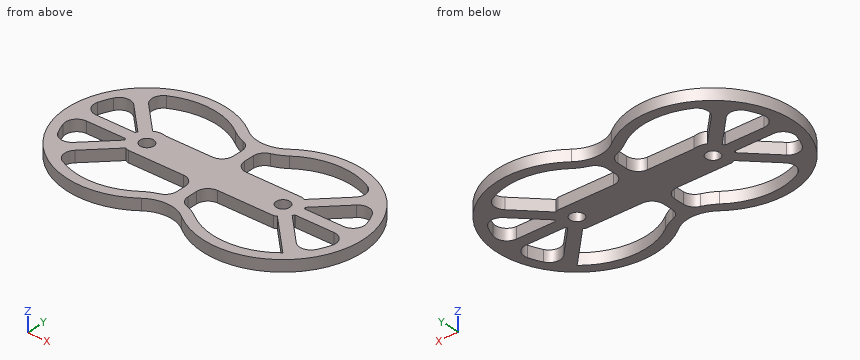
from build123d import *

# Parameters (mm, degrees)
SKETCH1_R           = 6
BOSS_EXTRUDE2_DEPTH = 10
FILLET2_R           = 10


with BuildPart() as part:
    # Sketch1 → Boss-Extrude2 (new body)
    with BuildSketch(Plane.XY):
        with BuildLine():
            ThreePointArc((-18.165151778, 55.726150839), (-130.527825355, 0), (-18.165151778, -55.726150839))
            ThreePointArc((-18.165151778, -55.726150839), (-0.527825355, -49.783359328), (17.109501067, -55.726150839))
            ThreePointArc((17.109501067, -55.726150839), (129.472174645, 0), (17.109501067, 55.726150839))
            ThreePointArc((17.109501067, 55.726150839), (-0.527825355, 49.783359328), (-18.165151778, 55.726150839))
        make_face()
        with Locations((-60.527825355, 0)):
            Circle(SKETCH1_R, mode=Mode.SUBTRACT)
        with Locations((59.472174645, 0)):
            Circle(SKETCH1_R, mode=Mode.SUBTRACT)
        with BuildLine():
            Line((-56.235975609, 14.912672635), (-5.527825355, 14.965504266))
            Line((-5.527825355, 14.965504266), (-5.527825355, 41.980686961))
            ThreePointArc((-5.527825355, 41.980686961), (-15.345309937, 44.512654742), (-24.210827936, 49.431643964))
            ThreePointArc((-24.210827936, 49.431643964), (-62.58583764, 61.303966527), (-100.078223296, 46.884728315))
            Line((-100.078223296, 46.884728315), (-67.337537784, 13.944016494))
            ThreePointArc((-67.337537784, 13.944016494), (-61.876707041, 15.459246345), (-56.235975609, 14.912672635))
        make_face(mode=Mode.SUBTRACT)
        with BuildLine():
            Line((-64.123905218, -15.095561897), (-5.527825355, -15.034512017))
            Line((-5.527825355, -15.034512017), (-5.527825355, -41.980686961))
            ThreePointArc((-5.527825355, -41.980686961), (-15.345309937, -44.512654742), (-24.210827936, -49.431643964))
            ThreePointArc((-24.210827936, -49.431643964), (-62.602390706, -61.303408593), (-100.103536918, -46.863362884))
            Line((-100.103536918, -46.863362884), (-67.345067046, -13.940336979))
            ThreePointArc((-67.345067046, -13.940336979), (-65.766427516, -14.607012931), (-64.123905218, -15.095561897))
        make_face(mode=Mode.SUBTRACT)
        with BuildLine():
            Line((-107.170792468, 39.835227443), (-74.430106955, 6.894515622))
            ThreePointArc((-74.430106955, 6.894515622), (-74.855512615, 5.960298411), (-75.218222877, 5))
            Line((-75.218222877, 5), (-121.6621997, 5))
            ThreePointArc((-121.6621997, 5), (-117.161402857, 23.559491206), (-107.170792468, 39.835227443))
        make_face(mode=Mode.SUBTRACT)
        with BuildLine():
            Line((-121.6621997, -5), (-75.218222877, -5))
            ThreePointArc((-75.218222877, -5), (-74.857121477, -5.956429468), (-74.433828207, -6.887006899))
            Line((-74.433828207, -6.887006899), (-107.192298079, -39.810032805))
            ThreePointArc((-107.192298079, -39.810032805), (-117.167762266, -23.544198292), (-121.6621997, -5))
        make_face(mode=Mode.SUBTRACT)
        with BuildLine():
            Line((4.472174645, 41.980686961), (4.472174645, 14.975923031))
            Line((4.472174645, 14.975923031), (63.304903434, 15.03721947))
            ThreePointArc((63.304903434, 15.03721947), (64.821395332, 14.56686711), (66.281887074, 13.944016494))
            Line((66.281887074, 13.944016494), (99.022572586, 46.884728315))
            ThreePointArc((99.022572586, 46.884728315), (61.530186929, 61.303966527), (23.155177226, 49.431643964))
            ThreePointArc((23.155177226, 49.431643964), (14.289659226, 44.512654742), (4.472174645, 41.980686961))
        make_face(mode=Mode.SUBTRACT)
        with BuildLine():
            Line((99.047886208, -46.863362884), (66.289416336, -13.940336979))
            ThreePointArc((66.289416336, -13.940336979), (64.962019266, -14.514454361), (63.586938832, -14.962502967))
            Line((63.586938832, -14.962502967), (4.472174645, -15.024093252))
            Line((4.472174645, -15.024093252), (4.472174645, -41.980686961))
            ThreePointArc((4.472174645, -41.980686961), (14.289659226, -44.512654742), (23.155177226, -49.431643964))
            ThreePointArc((23.155177226, -49.431643964), (61.546739995, -61.303408593), (99.047886208, -46.863362884))
        make_face(mode=Mode.SUBTRACT)
        with BuildLine():
            Line((106.136647368, -39.810032805), (73.378177497, -6.887006899))
            ThreePointArc((73.378177497, -6.887006899), (73.801470767, -5.956429468), (74.162572167, -5))
            Line((74.162572167, -5), (120.606548989, -5))
            ThreePointArc((120.606548989, -5), (116.112111556, -23.544198292), (106.136647368, -39.810032805))
        make_face(mode=Mode.SUBTRACT)
        with BuildLine():
            Line((120.606548989, 5), (74.162572167, 5))
            ThreePointArc((74.162572167, 5), (73.799861904, 5.960298411), (73.374456245, 6.894515622))
            Line((73.374456245, 6.894515622), (106.115141757, 39.835227443))
            ThreePointArc((106.115141757, 39.835227443), (116.105752147, 23.559491206), (120.606548989, 5))
        make_face(mode=Mode.SUBTRACT)
    extrude(amount=BOSS_EXTRUDE2_DEPTH)

    # Fillet2
    fillet2_edges = [part.edges().sort_by_distance(p)[0] for p in [
        (4.472174645, -15.024093252, 5),
        (4.472174645, -41.980686961, 5),
        (106.136647368, -39.810032805, 5),
        (120.606548989, -5, 5),
        (120.606548989, 5, 5),
        (106.115141757, 39.835227443, 5),
        (-100.103536918, -46.863362884, 5),
        (-5.527825355, -41.980686961, 5),
        (-5.527825355, -15.034512017, 5),
        (-121.6621997, -5, 5),
        (-107.192298079, -39.810032805, 5),
        (-107.170792468, 39.835227443, 5),
        (-121.6621997, 5, 5),
        (-5.527825355, 14.965504266, 5),
        (-5.527825355, 41.980686961, 5),
        (-100.078223296, 46.884728315, 5),
        (99.022572586, 46.884728315, 5),
        (4.472174645, 41.980686961, 5),
        (4.472174645, 14.975923031, 5),
    ]]
    fillet(fillet2_edges, radius=FILLET2_R)


solid = part.part
Part model, mm, in its own coordinate system. Coordinates: 2 decimals unless noted, no trailing zeros. Loops run counter-clockwise (first coordinate to the right, second up) from the corner with the lowest first, then second, coordinate; pieces in that order, holes last. Notation, with made-up numbers: M -7,-28.75 L 31,-28.75 A21 cw 31,-6.75 Z; hole C 22.25,22.5 d7. An arc over 180 degrees is marked long. Use a Markdown table: item, result. Add a question column.
Q1. Cut at C-C (z = 6.5). Give the number of separate pieces and of enclosed holes in the cut face, and give its area (3 significant figures).
Q2. Cut at B-B (x = -9.5). Write the cut outline in (y, z), and give its area (3 significant figures).
Q3. Cut at A-A (y = 0). Write the cut outline in (x, z).
Q4. Pin check, flat tips, straight feed: P1, Ø1.5, axis at x = -8.5, z = 5, coming from the +Y side; P2, Ø5, axis at x = 42.5, z = 7.5, coming from the +Y side; P3, Ø15.5, axis at x = 59.47, y = 0, coming from the -Z side; P4, Ø2, axis at x = -29, z = 4.5, coming from the +Y side. Stop position of each tip, or through.
Q5. Probe L1, parallel to X at y = -16, z = 3.25; L2, parallel to X at y = 53.5, z = 4.5; L3, parallel to Y at x = -58, z = 6. List the from-to ranges inside material, lowest first.
Worked out:
| question | item | result |
|---|---|---|
| 1 | separate pieces | 1 |
| 1 | enclosed holes | 10 |
| 1 | area | 13,700 mm2 |
| 2 | outline | M -51.2,0 L -41.95,0 L -41.95,10 L -51.2,10 Z; M -17.07,0 L 16.98,0 L 16.98,10 L -17.07,10 Z; M 41.95,0 L 51.2,0 L 51.2,10 L 41.95,10 Z |
| 2 | area | 525 mm2 |
| 3 | outline | M -130.53,0 L -66.53,0 L -66.53,10 L -130.53,10 Z; M -54.53,0 L 53.47,0 L 53.47,10 L -54.53,10 Z; M 65.47,0 L 129.47,0 L 129.47,10 L 65.47,10 Z |
| 4 | P1 | stops at y = 51.12 |
| 4 | P2 | stops at y = 68.49 |
| 4 | P3 | stops at z = 0 |
| 4 | P4 | stops at y = 62.99 |
| 5 | L1 | x = -128.67 to -119.58, -83.5 to -69.39, -11.26 to 10.14, 68.34 to 82.45, 118.52 to 127.62 |
| 5 | L2 | x = -105.67 to -90.36, -30.53 to -14.77, 13.71 to 29.47, 89.31 to 104.61 |
| 5 | L3 | y = -69.95 to -61.29, -15.09 to -5.44, 5.44 to 15.31, 61.29 to 69.95 |
